Input: part model. Units: mm. Frame: model coordinates. A direction names the side the tool comes from. Coordinates: 2 decimals unless noted, no trailing zeros. Write each loop counter-clockwise with the first axis right and the second up, starting at its lowest first coordinate (ties: lowest second). Pieces come first, ordered by that corner, then holes.
1) Line query: L1, parallel to Y at x = -1.7, z = -0.7; L2, parallel to Y at x = 8.5, z = 13.5; L3, parallel to X at y = 25.5, z = 9.5. Output: solid intervals per line, ascending.
2) Section query D-D (z = 17.25). Output: boundary loops of the cut face in (x, y), then the cut area to 3 significant figures.
3) Pin query (flat end, axial travel): pin 1 Ø2 at (x, z) = (19.5, -1) entering from -Y; pin 2 Ø2 at (y, z) = (34.5, 6.5) entering from -X; pin 3 Ø5 at (x, y) = (6, 10.5) entering from +Z. Return the tip coordinate at first contact, or that it passes through.
4) Set-up query: faces 1 (the flat face through (6, 33, 6)), 2 (the flat face through (9, 0, 15)), 3 (the flat face through (2, 18, 6)). Return all of +Z, -Z, +X, -X, +Y, -Y with unobstructed straight access to the full face (end or side cutting, diameter ignored); none if empty.
5) Section query C-C (x = -1.75). Output: boundary loops of the cut face in (y, z), then the cut area to 3 significant figures.
6) Section query A-A (z = 4.5). Output: boundary loops of the cut face in (x, y).
7) Draft query along X for faces 4 (the flat face through (17, 33, 6)), 5 (the cylindrical face through (5.55, -12.3, 8.35)), 6 (the flat face through (3, 36.5, 6)), 7 (the cylindrical face through (17.15, 36.44, -0.99)). Return one class per face: pulls with the +X half, pulls with the -X half, needs draft (parallel to the pull), parting line crosses it, or undercut.
8) Section query B-B (y = 12). Output: boundary loops of the cut face in (x, z), then the cut area to 3 significant figures.
from build123d import *

# Parameters (mm, degrees)
SKETCH_R          = 1.55
PAD_DEPTH         = 12
SKETCH001_W       = 30
SKETCH001_H       = 50
SKETCH001_R       = 1.6
PAD001_DEPTH      = 2
SKETCH002_W       = 4
SKETCH002_H       = 7
POCKET_DEPTH      = 12
SKETCH004_R       = 4
PAD002_DEPTH      = 19
PAD002_DEPTH_BACK = 2


with BuildPart() as part:
    # Sketch → Pad (new body)
    with BuildSketch(Plane.XY):
        Polygon((0, 0), (17, 0), (17, 7), (2, 7), (2, 29.5), (17, 29.5), (17, 36.5), (0, 36.5), align=None)
        with Locations((12, 33)):
            Circle(SKETCH_R, mode=Mode.SUBTRACT)
        with Locations((12, 3.5)):
            Circle(SKETCH_R, mode=Mode.SUBTRACT)
    extrude(amount=PAD_DEPTH)

    # Sketch001 → Pad001 (join)
    with BuildSketch(Plane.XY):
        with Locations((8.5, 25)):
            Rectangle(SKETCH001_W, SKETCH001_H)
        with Locations((-1.7, 38)):
            Circle(SKETCH001_R, mode=Mode.SUBTRACT)
        with Locations((-1.7, 12)):
            Circle(SKETCH001_R, mode=Mode.SUBTRACT)
        with Locations((17.5, 12)):
            Circle(SKETCH001_R, mode=Mode.SUBTRACT)
        with Locations((17.5, 38)):
            Circle(SKETCH001_R, mode=Mode.SUBTRACT)
    extrude(amount=-PAD001_DEPTH)

    # Sketch002 (on DatumPlane) → Pocket (cut)
    with BuildSketch(Plane.XY.offset(12)):
        with Locations((8, 33)):
            Rectangle(SKETCH002_W, SKETCH002_H)
    extrude(amount=-POCKET_DEPTH, mode=Mode.SUBTRACT)

    # Sketch004 → Pad002 (join, two sides)
    with BuildSketch(Plane.XY) as pad002_sk:
        with BuildLine():
            ThreePointArc((0, -15), (8.5, -23.5), (17, -15))
            Line((17, -15), (17, 0))
            Line((17, 0), (0, 0))
            Line((0, 0), (0, -15))
        make_face()
        with Locations((8.5, -15)):
            Circle(SKETCH004_R, mode=Mode.SUBTRACT)
    extrude(amount=PAD002_DEPTH)
    extrude(pad002_sk.sketch, amount=-PAD002_DEPTH_BACK)


solid = part.part
Answer:
1. L1: y = 0 to 10.4, 13.6 to 36.4, 39.6 to 50
1. L2: y = -23.5 to -19, -11 to 0
1. L3: x = 0 to 2
2. outline: (0, -15) arc R8.5 ccw to (17, -15) - (17, 0) - (0, 0) - close; hole circle Ø8 at (8.5, -15)
2. area: 318 mm2
3. pin 1: stops at y = 0
3. pin 2: stops at x = 0
3. pin 3: stops at z = 0
4. face 1: +Z, +Y
4. face 2: +Z, +X, -X, +Y
4. face 3: +Z, +X
5. outline: (0, -2) - (10.4, -2) - (10.4, 0) - (0, 0) - close; (13.6, -2) - (36.4, -2) - (36.4, 0) - (13.6, 0) - close; (39.6, -2) - (50, -2) - (50, 0) - (39.6, 0) - close
5. area: 87.2 mm2
6. outline: (0, -15) arc R8.5 ccw to (17, -15) - (17, 7) - (2, 7) - (2, 29.5) - (6, 29.5) - (6, 36.5) - (0, 36.5) - close; (10, 29.5) - (17, 29.5) - (17, 36.5) - (10, 36.5) - close; hole circle Ø8 at (8.5, -15); hole circle Ø3.1 at (12, 3.5); hole circle Ø3.1 at (12, 33)
7. face 4: pulls with the +X half
7. face 5: undercut
7. face 6: needs draft
7. face 7: undercut
8. outline: (-6.5, -2) - (-3.3, -2) - (-3.3, 0) - (-6.5, 0) - close; (-0.1, -2) - (15.9, -2) - (15.9, 0) - (2, 0) - (2, 12) - (0, 12) - (0, 0) - (-0.1, 0) - close; (19.1, -2) - (23.5, -2) - (23.5, 0) - (19.1, 0) - close
8. area: 71.2 mm2
